Answer from the drawing. Dimensions are ordinates in mm from the lowest x, y and z of the part. Coordinates: 2 decimals unless noted, no trailing zeros. Write each loop counter-clockwise with the first axis right and the second up, starting at its lowest first coordinate (ties: lowest second). Pieces come first, ordered by that corner, then holes. Notation, with made-up numbers: (49.25, 66.5) -> (81.25, 66.5) arc R16 cw to (81.25, 91.5) -> close; hole circle Ø2 at (51, 62). An arc over 180 degrees is marked (long way). Answer as a JSON object with one key per item and string values. Group by question number.
(1) Find section C-C (z = 214). Give the vertices of the cut face in (x, y), then the cut area to 3 significant figures.
(2) Find section A-A (x = 133). Give the vertices of the cut face in (y, z), then the cut area to 3 significant figures.
(3) Flat-ended cylindrical pins translate along their axes: P1, Ø12, axis at x = 148, z = 165.5, coming from the -Y side; P2, Ø4, axis at y = 13, z = 59.5, coming from the +X side; P3, Ø2, axis at y = 35.5, z = 253, coming from the -X side. Find the tip coordinate at first contact, or state that the pin passes through.
(4) Find section B-B (y = 13). Give the vertices of the cut face in (x, z).
(5) Straight lines are drawn through the part: L1, parallel to Y at x = 376, z = 291; L2, parallel to Y at x = 31, z = 96; L3, parallel to X at y = 18.5, z = 122. For each, find the intervals that lie inside material, in ascending order.
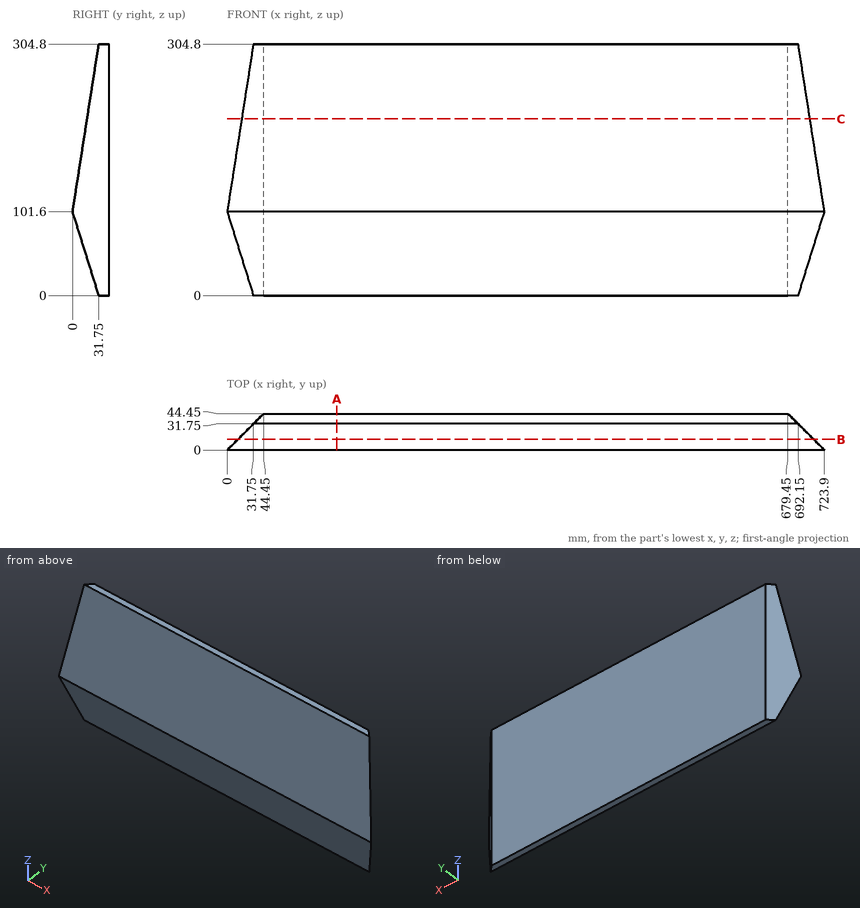
Results below:
{
 "1": {"outline": "(17.56, 17.56) -> (706.34, 17.56) -> (679.45, 44.45) -> (44.45, 44.45) -> close", "area": "17,800 mm2"},
 "2": {"outline": "(0, 101.6) -> (31.75, 0) -> (44.45, 0) -> (44.45, 304.8) -> (31.75, 304.8) -> close", "area": "8,710 mm2"},
 "3": {"P1": "stops at y = 9.05", "P2": "stops at x = 711.35", "P3": "stops at x = 34.5"},
 "4": {"outline": "(13, 60) -> (710.9, 60) -> (710.9, 184.8) -> (13, 184.8) -> close"},
 "5": {"L1": "y = 29.59 to 44.45", "L2": "y = 1.75 to 31", "L3": "x = 18.5 to 705.4"}
}
